The model under review builds one solid part; all positions refer to its coordinate system, in mm. Round coordinates to 2 decimals unless told otherwise and drop trailing zeros. Write each loop counter-clockwise with the first axis right and the second up, starting at its lowest first coordinate (ties: lowest second). Pieces come first, ordered by that corner, then holes. Notation, with made-up numbers: (39.5, 89) - (85.5, 89) arc R14 ccw to (85.5, 111) - close; hole circle Ø3 at (29, 14). An arc over 180 degrees is marked (long way). Write each question's results on one line, items separated by ' | '.
```python
from build123d import *

# Parameters (mm, degrees)
SKETCH1_W           = 40
SKETCH1_H           = 20
BOSS_EXTRUDE1_DEPTH = 70
CUT_EXTRUDE1_DEPTH  = 40


with BuildPart() as part:
    # Sketch1 → Boss-Extrude1 (new body)
    with BuildSketch(Plane(origin=(0, 0, 0), x_dir=(1, 0, 0), z_dir=(0, 1, 0))):
        with Locations((20, 10)):
            Rectangle(SKETCH1_W, SKETCH1_H)
    extrude(amount=BOSS_EXTRUDE1_DEPTH)

    # Sketch2 → Cut-Extrude1 (cut)
    with BuildSketch(Plane(origin=(0, 0, 0), x_dir=(0, 0, -1), z_dir=(1, 0, 0))):
        Polygon((10, 70), (20, 49.892008703), (27.740621585, 66.282102968), (20, 74.973147169), align=None)
    extrude(amount=CUT_EXTRUDE1_DEPTH, mode=Mode.SUBTRACT)


solid = part.part
```
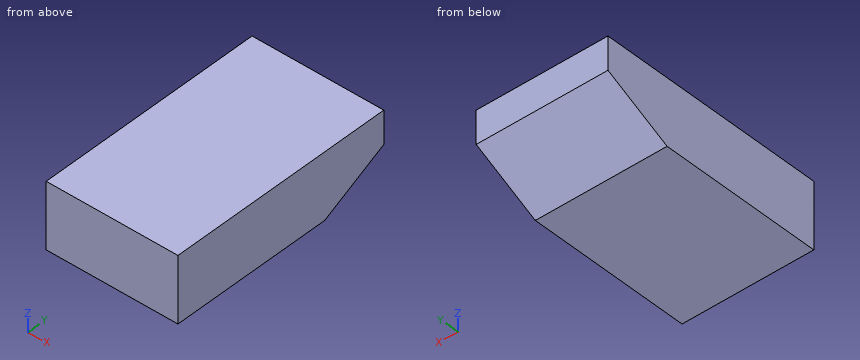
Q1. We need section C-C (y = 51.5). State the section outline as (x, z) points.
Evaluation:
outline: (0, -19.2) - (40, -19.2) - (40, 0) - (0, 0) - close
Q2. For probe 1 along Y at (x, z) = (26.5, -15.25); probe 2 along Y at (x, z) = (15, -13); probe 3 along Z at (x, y) = (15.5, 66.5), list the stretches that pass through material, from the lowest coordinate up.
Evaluation:
probe 1: y = 0 to 59.44 | probe 2: y = 0 to 63.97 | probe 3: z = -11.74 to 0
Q3. We need section B-B (z = -17.75). State the section outline as (x, y) points, plus the area to 3 significant figures.
Evaluation:
outline: (0, 0) - (40, 0) - (40, 54.42) - (0, 54.42) - close | area: 2,180 mm^2
Q4. Insertion check: P1, Ø12, axis at x = 34, y = 17.5, coming from the +Z side; P2, Ø4, axis at x = 18, z = -17, coming from the +Y side. Each pin has a flat end and moves straight along its axis. Give the tip position at first contact, or say it passes through.
Evaluation:
P1: stops at z = 0 | P2: stops at y = 59.95
Q5. We need section A-A (x = 5). State the section outline as (y, z) points, plus the area to 3 significant figures.
Evaluation:
outline: (0, -20) - (49.89, -20) - (70, -10) - (70, 0) - (0, 0) - close | area: 1,300 mm^2
